Verification items for the finished model (mm, model axes). A direction names the side the tool comes from. Coordinates: 2 decimals unless noted, no trailing zeros. Loops run counter-clockwise (first coordinate to the right, second up) from the corner with the lowest first, then second, coordinate; pieces in that order, holes last. Notation, with made-up numbers: (-28, 19) -> (15, 19) arc R20 ccw to (15, 41) -> close; hole circle Ø3 at (-12.75, 70.5). An arc over 180 degrees is marked (long way). Write item = value, one per line.
```python
from build123d import *

# Parameters (mm, degrees)
SKETCH2_W           = 0.4
SKETCH2_H           = 2
BOSS_EXTRUDE1_DEPTH = 5.8
CHAMFER1_SIZE       = 0.3
SKETCH3_R           = 7
BOSS_EXTRUDE2_DEPTH = 0.5
SKETCH4_R           = 5.7
SKETCH4_R_2         = 4.75
CUT_EXTRUDE1_DEPTH  = 0.5
FILLET1_R           = 0.1
FILLET2_R           = 0.1
BOSS_EXTRUDE3_START = 1
SKETCH5_R           = 8
BOSS_EXTRUDE3_DEPTH = 1
CHAMFER2_SIZE       = 0.3


with BuildPart() as part:
    # Sketch1 → Revolve1 (revolve)
    with BuildSketch(Plane.XY, mode=Mode.PRIVATE) as revolve1_sk:
        Polygon((0, 14.75), (-7.5, 14.75), (-8.9, 12.75), (-8, 12.75), (-8, -12.85), (-7, -12.85), (-7, -14.75), (0, -14.75), align=None)
    revolve(revolve1_sk.sketch.rotate(Axis((0, 14.75, 0), (0, -1, 0)), 270), axis=Axis((0, 14.75, 0), (0, -1, 0)))

    # Sketch2 → Boss-Extrude1 (add)
    with BuildSketch(Plane.XZ.offset(14.75)):
        with Locations((-5.2, 0)):
            Rectangle(SKETCH2_W, SKETCH2_H)
        Polygon((-0.717635253, 5.444722182), (-0.594028456, 5.064299576), (-2.496141488, 4.446265587), (-2.619748286, 4.826688194), align=None)
        Polygon((4.956477022, 2.365023368), (4.632870224, 2.129909267), (3.45729972, 3.747943256), (3.780906517, 3.983057357), align=None)
        Polygon((3.780906517, -3.983057357), (3.45729972, -3.747943256), (4.632870224, -2.129909267), (4.956477022, -2.365023368), align=None)
        Polygon((-2.619748286, -4.826688194), (-2.496141488, -4.446265587), (-0.594028456, -5.064299576), (-0.717635253, -5.444722182), align=None)
    extrude(amount=BOSS_EXTRUDE1_DEPTH)

    # Chamfer1
    chamfer1_edges = [part.edges().sort_by_distance(p)[0] for p in [
        (-5.2, -20.55, -1),
        (-5.2, -20.55, 1),
        (-2.557944887, -20.55, 4.63647689),
        (-0.655831854, -20.55, 5.254510879),
        (3.619103118, -20.55, 3.865500306),
        (4.794673623, -20.55, 2.247466318),
        (4.794673623, -20.55, -2.247466318),
        (3.619103118, -20.55, -3.865500306),
        (-0.655831854, -20.55, -5.254510879),
        (-2.557944887, -20.55, -4.63647689),
    ]]
    chamfer(chamfer1_edges, length=CHAMFER1_SIZE)

    # Sketch3 → Boss-Extrude2 (add)
    with BuildSketch(Plane(origin=(0, 14.75, 0), x_dir=(1, 0, 0), z_dir=(0, 1, 0))):
        with Locations(Location((0, 0, 0), (0, 0, 270))):
            Circle(SKETCH3_R)
    extrude(amount=BOSS_EXTRUDE2_DEPTH)

    # Sketch4 → Cut-Extrude1 (cut)
    with BuildSketch(Plane(origin=(0, 15.25, 0), x_dir=(1, 0, 0), z_dir=(0, 1, 0))):
        with Locations(Location((0, 0, 0), (0, 0, 270))):
            Circle(SKETCH4_R)
        with Locations(Location((0, 0, 0), (0, 0, 270))):
            Circle(SKETCH4_R_2, mode=Mode.SUBTRACT)
    extrude(amount=-CUT_EXTRUDE1_DEPTH, mode=Mode.SUBTRACT)

    # Fillet1
    fillet1_edges = [part.edges().sort_by_distance(p)[0] for p in [
        (0, 15.25, -7),
        (0, 15.25, -4.75),
    ]]
    fillet(fillet1_edges, radius=FILLET1_R)

    # Fillet2
    fillet2_edges = [part.edges().sort_by_distance(p)[0] for p in [
        (0, 12.75, -8.9),
    ]]
    fillet(fillet2_edges, radius=FILLET2_R)

    # Sketch5 → Boss-Extrude3 (add)
    with BuildSketch(Plane(origin=(0, 10.75, 0), x_dir=(-1, 0, 0), z_dir=(0, -1, 0)).offset(BOSS_EXTRUDE3_START)):
        Polygon((0, 10.969655115), (-9.5, 5.484827557), (-9.5, -5.484827557), (0, -10.969655115), (9.5, -5.484827557), (9.5, 5.484827557), align=None)
        with Locations(Location((0, 0, 0), (0, 0, 270))):
            Circle(SKETCH5_R, mode=Mode.SUBTRACT)
    extrude(amount=-BOSS_EXTRUDE3_DEPTH)

    # Chamfer2
    chamfer2_edges = [part.edges().sort_by_distance(p)[0] for p in [
        (-4.75, 9.75, -8.227241336),
        (4.75, 9.75, -8.227241336),
        (9.5, 9.75, 0),
        (4.75, 9.75, 8.227241336),
        (-4.75, 9.75, 8.227241336),
        (-9.5, 9.75, 0),
        (-4.75, 10.75, -8.227241336),
        (4.75, 10.75, -8.227241336),
        (9.5, 10.75, 0),
        (4.75, 10.75, 8.227241336),
        (-4.75, 10.75, 8.227241336),
        (-9.5, 10.75, 0),
    ]]
    chamfer(chamfer2_edges, length=CHAMFER2_SIZE)


solid = part.part
```
1) Depth check by flat-ended pin: pin 1 Ø8 at (y, z) = (4, 5.5) entering from +X; pin 2 Ø5 at (x, y) = (3, 1) entering from +Z; pin 3 Ø3 at (x, y) = (-3, -12.5) entering from +Z. Enter the tip coordinate at first touch or a pass-through.
Ans:
pin_1 = 7.86
pin_2 = 7.98
pin_3 = 7.86
2) Material ranges on line 1 (X direction, y = 15, z = 0); line 2 (Y direction, x = -4.5, z = -8); line 3 (Y direction, x = 4.5, z = -1), recorded low to high.
Ans:
line_1 = -7 to -5.7, -4.75 to 4.75, 5.7 to 7
line_2 = 9.75 to 10.75
line_3 = -14.75 to 15.25
3) Release check for a two-part mould opening along Z. For faces 4 (the face through (-4.607, 9.898, 8.134)), 5 (the face through (0, -14.75, 0)), 6 (the face through (-2, 9.75, 8)) record: pulls with the +Z half, pulls with the -Z half, needs draft (parallel to the pull), parting line crosses it, or undercut.
Ans:
face_4 = pulls with the +Z half
face_5 = undercut
face_6 = needs draft
4) Tool access check on faces 1 (the face through (-1.53, -17.61, 4.76)), 2 (the face through (5, 14.75, -1)), 3 (the face through (6, -12.85, 4)). Record the directions out of +Z, -Z, +X, -X, +Y, -Y that give a thin tool (end or side, any length) a straight path to the whole face; none if there is none.
Ans:
face_1 = +X, -Y
face_2 = +Y
face_3 = -Y
5) Sectioned sample at A-A, the plane y = -7.5. Record the cut outline in (x, z).
Ans:
outline = circle Ø16 at (0, 0)
